Check sheet for the modelled part. Datum: model origin and axes. Units: mm. Give positions to 0.01 mm unless a question says otherwise; leave off trailing zeros. Write each loop counter-clockwise with the first axis right and the second up, starting at its lowest first coordinate (ties: lowest second). Pieces come first, ordered by that corner, then holes. Notation, with made-up numbers: M 76.5,87 L 122.5,87 A23 cw 122.5,109 Z; hole C 37.5,6 d11. An arc over 180 degrees is marked long. Write each question's results on one line, items separated by ' | '. Start each with the question number.
from build123d import *

# Parameters (mm, degrees)
F0_R      = 57.9627661604
F1_DEPTH  = 25.4
F2_R      = 32.9835616542
F1_FACE_R = 57.9627661604
F3_DEPTH  = 25.4
F4_R      = 57.9627661604
F5_DEPTH  = 25.4


with BuildPart() as f1:
    # F0 (on Top) → F1 (new body)
    with BuildSketch(Plane.XY):
        Circle(F0_R)
    extrude(amount=F1_DEPTH)

    # F2 (on Top) + F1_face (on face) → F3 (join)
    with BuildSketch(Plane.XY):
        Circle(F2_R)
    with BuildSketch(Plane(origin=(0, 0, 0), x_dir=(1, 0, 0), z_dir=(0, 0, -1))):
        Circle(F1_FACE_R)
    extrude(amount=F3_DEPTH, dir=(0, 0, 1))

    # F4 (on Top) → F5 (join)
    with BuildSketch(Plane.XY):
        Circle(F4_R)
    extrude(amount=F5_DEPTH)


solid = f1.part
Q1. Scan lines: L1, parallel to Y at x = -1.5, z = 9.5; L2, parallel to X at y = 4.5, z = 20.75; L3, parallel to X at y = 19, z = 5.75. Record each from-to range of solid material in increasing order.
Q2. Section check B-B on x = 25. Record the boundary of the cut face in (y, z).
Q3. Section check A-A on z = 12.75. Record the boundary of the cut face in (x, y).
Q4. Section check C-C on y = 32. Record the boundary of the cut face in (x, z), plus the area to 3 significant figures.
Q5. Depth check by flat-ended pin: pin 1 Ø10 at (y, z) = (20.5, 18) entering from +X; pin 2 Ø10 at (y, z) = (38.5, 8) entering from +X; pin 3 Ø2 at (x, z) = (-2, 19.5) entering from -Y. Enter the tip coordinate at first touch or a pass-through.
Check result:
1) L1: -57.94 to 57.94 | L2: -57.79 to 57.79 | L3: -54.76 to 54.76
2) outline: M -52.29,0 L 52.29,0 L 52.29,25.4 L -52.29,25.4 Z
3) outline: C 0,0 d115.93
4) outline: M -48.33,0 L 48.33,0 L 48.33,25.4 L -48.33,25.4 Z | area: 2,460 mm^2
5) pin 1: x = 55.85 | pin 2: x = 47.3 | pin 3: y = -57.95
